from build123d import *

# Parameters (mm, degrees)
F0_W     = 210
F0_H     = 225
F1_DEPTH = 25
F3_DEPTH = 95


with BuildPart() as f1:
    # F0 (on Top) → F1 (new body)
    with BuildSketch(Plane.XY):
        Rectangle(F0_W, F0_H)
    extrude(amount=F1_DEPTH)

    # F2 (on face) → F3 (join)
    with BuildSketch(Plane.XY.offset(25)):
        with BuildLine():
            Line((-71, -32.5), (-71, -112.5))
            Line((-71, -112.5), (-56, -112.5))
            Line((-56, -112.5), (-56, -46.481817))
            ThreePointArc((-56, -46.481817), (7.488853, -14.988853), (38.981817, 48.5))
            Line((38.981817, 48.5), (105, 48.5))
            Line((105, 48.5), (105, 63.5))
            Line((105, 63.5), (25, 63.5))
            ThreePointArc((25, 63.5), (-3.117749, -4.382251), (-71, -32.5))
        make_face()
    extrude(amount=F3_DEPTH)


solid = f1.part
Input: part model. Units: mm. Frame: model coordinates. A direction names the side the tool comes from. Give positions to 0.01 mm unless a question says otherwise; leave off trailing zeros. Write each loop counter-clockwise with the first axis right and the second up, starting at its lowest first coordinate (ties: lowest second). Pieces come first, ordered by that corner, then holes.
Q1. Section A-A, the plane x = 72. Output: boundary loops of the cut face in (y, z), plus the area to 3 significant figures.
Q2. First-contact query: P1, Ø6, axis at y = 43.5, z = 48.5, coming from the -X side; P2, Ø1.5, axis at x = -46.5, y = -9, coming from the -Z side; P3, Ø1.5, axis at x = 46, z = 52.5, coming from the +Y side; P4, Ø12, axis at x = 31, y = -58, coming from the +Z side. Flat tips, straight axial feed; report the tip coordinate or a pass-through.
Q3. Section C-C, the plane y = 85. Output: boundary loops of the cut face in (x, z).
Q4. Section B-B, the plane y = -92. Output: boundary loops of the cut face in (x, z).
Q5. Material intervals for probe 1 along Y at (x, z) = (85, 59); probe 2 along Z at (x, y) = (74.5, 35); probe 3 along X at (y, z) = (-92.5, 67.5), sorted ascending.
Q6. Set-up query: faces 1 (the face through (-56, -80, 72)), 2 (the face through (-2.375, -3.632, 71.835)), 3 (the face through (105, 8, 24)), 4 (the face through (66, 63.5, 72)), 5 (the face through (-71, -72, 72)). Return all of +Z, -Z, +X, -X, +Y, -Y with unobstructed straight access to the full face (end or side cutting, diameter ignored); none if empty.
Filled in:
1. outline: (-112.5, 0) - (112.5, 0) - (112.5, 25) - (63.5, 25) - (63.5, 120) - (48.5, 120) - (48.5, 25) - (-112.5, 25) - close
1. area: 7,050 mm2
2. P1: stops at x = 22.2
2. P2: stops at z = 0
2. P3: stops at y = 63.5
2. P4: stops at z = 25
3. outline: (-105, 0) - (105, 0) - (105, 25) - (-105, 25) - close
4. outline: (-105, 0) - (105, 0) - (105, 25) - (-56, 25) - (-56, 120) - (-71, 120) - (-71, 25) - (-105, 25) - close
5. probe 1: y = 48.5 to 63.5
5. probe 2: z = 0 to 25
5. probe 3: x = -71 to -56
6. face 1: +Z, +X, -Y
6. face 2: +Z, -X, +Y
6. face 3: +Z, -Z, +X, +Y, -Y
6. face 4: +Z, +X, -X, +Y
6. face 5: +Z, -X, +Y, -Y
